The model under review builds one solid part; all positions refer to its coordinate system, in mm. Face numbers are marked on the shaded views. A direction names the side the tool comes from. Give positions to 0.01 mm unless a question says otherwise; leave off trailing zeros. Write each loop counter-clockwise with the first axis right and the second up, starting at its lowest first coordinate (ties: lowest second). Pieces come first, ordered by that corner, then holes. Notation, with made-up numbers: M 85.5,-11.5 L 96.5,-11.5 A25 ccw 96.5,3.5 Z; hole C -9.5,47 d3. An arc over 180 degrees is marked long. Write item = value, one per line. Start each with the question number.
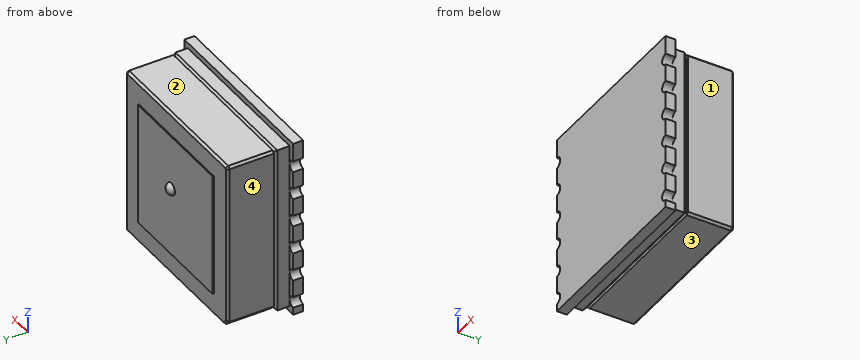
```python
from build123d import *

# Parameters (mm, degrees)
EXTRUDE1_DEPTH = 0.9
SKETCH2_W      = 15
SKETCH2_H      = 15
EXTRUDE2_DEPTH = 1.4
CHAMFER1_SIZE  = 0.3
SKETCH3_W      = 15
SKETCH3_H      = 15
EXTRUDE3_DEPTH = 4.15
CHAMFER2_SIZE  = 0.5
CHAMFER3_SIZE  = 0.2
CHAMFER4_SIZE  = 0.2
SKETCH4_R      = 0.55
EXTRUDE4_DEPTH = 0.5
FILLET1_R      = 0.5
SKETCH5_W      = 11
SKETCH5_H      = 11
EXTRUDE5_DEPTH = 0.1


with BuildPart() as part:
    # Sketch1 → Extrude1 (new body)
    with BuildSketch(Plane(origin=(0, 0, 0), x_dir=(1, 0, 0), z_dir=(0, 1, 0))):
        with BuildLine():
            Line((8, 6.35), (8, 4.81))
            ThreePointArc((8, 4.81), (7.5, 4.31), (8, 3.81))
            Line((8, 3.81), (8, 2.27))
            ThreePointArc((8, 2.27), (7.5, 1.77), (8, 1.27))
            Line((8, 1.27), (8, -0.27))
            ThreePointArc((8, -0.27), (7.5, -0.77), (8, -1.27))
            Line((8, -1.27), (8, -2.81))
            ThreePointArc((8, -2.81), (7.5, -3.31), (8, -3.81))
            Line((8, -3.81), (8, -5.35))
            ThreePointArc((8, -5.35), (7.5, -5.85), (8, -6.35))
            Line((8, -6.35), (8, -8))
            Line((8, -8), (-8, -8))
            Line((-8, -8), (-8, -6.35))
            ThreePointArc((-8, -6.35), (-7.5, -5.85), (-8, -5.35))
            Line((-8, -5.35), (-8, -3.81))
            ThreePointArc((-8, -3.81), (-7.5, -3.31), (-8, -2.81))
            Line((-8, -2.81), (-8, -1.27))
            ThreePointArc((-8, -1.27), (-7.5, -0.77), (-8, -0.27))
            Line((-8, -0.27), (-8, 1.27))
            ThreePointArc((-8, 1.27), (-7.5, 1.77), (-8, 2.27))
            Line((-8, 2.27), (-8, 3.81))
            ThreePointArc((-8, 3.81), (-7.5, 4.31), (-8, 4.81))
            Line((-8, 4.81), (-8, 6.35))
            ThreePointArc((-8, 6.35), (-7.5, 6.85), (-8, 7.35))
            Line((-8, 7.35), (-8, 8))
            Line((-8, 8), (8, 8))
            Line((8, 8), (8, 7.35))
            ThreePointArc((8, 7.35), (7.5, 6.85), (8, 6.35))
        make_face()
    extrude(amount=EXTRUDE1_DEPTH)

    # Sketch2 → Extrude2 (add)
    with BuildSketch(Plane(origin=(0, 0.9, 0), x_dir=(1, 0, 0), z_dir=(0, 1, 0))):
        Rectangle(SKETCH2_W, SKETCH2_H)
    extrude(amount=EXTRUDE2_DEPTH)

    # Chamfer1
    chamfer1_edges = [part.edges().sort_by_distance(p)[0] for p in [
        (-7.5, 2.3, 0),
        (0, 2.3, 7.5),
        (7.5, 2.3, 0),
        (0, 2.3, -7.5),
    ]]
    chamfer(chamfer1_edges, length=CHAMFER1_SIZE)

    # Sketch3 → Extrude3 (add)
    with BuildSketch(Plane(origin=(0, 2.3, 0), x_dir=(1, 0, 0), z_dir=(0, 1, 0))):
        Rectangle(SKETCH3_W, SKETCH3_H)
    extrude(amount=EXTRUDE3_DEPTH)

    # Chamfer2
    chamfer2_edges = [part.edges().sort_by_distance(p)[0] for p in [
        (-7.5, 4.375, -7.5),
    ]]
    chamfer(chamfer2_edges, length=CHAMFER2_SIZE)

    # Chamfer3
    chamfer3_edges = [part.edges().sort_by_distance(p)[0] for p in [
        (-7.5, 4.375, 7.5),
        (7.5, 4.375, 7.5),
        (7.5, 4.375, -7.5),
    ]]
    chamfer(chamfer3_edges, length=CHAMFER3_SIZE)

    # Chamfer4
    chamfer4_edges = [part.edges().sort_by_distance(p)[0] for p in [
        (-7.5, 6.45, 0.15),
        (-7.25, 6.45, -7.25),
        (0.15, 6.45, -7.5),
        (7.5, 6.45, 0),
        (0, 6.45, 7.5),
        (-7.4, 6.45, 7.4),
        (7.4, 6.45, 7.4),
        (7.4, 6.45, -7.4),
    ]]
    chamfer(chamfer4_edges, length=CHAMFER4_SIZE)

    # Sketch4 → Extrude4 (add)
    with BuildSketch(Plane(origin=(0, 6.45, 0), x_dir=(1, 0, 0), z_dir=(0, 1, 0))):
        with Locations(Location((0.6, -0.63, 0), (0, 0, 270))):
            Circle(SKETCH4_R)
    extrude(amount=EXTRUDE4_DEPTH)

    # Fillet1
    fillet1_edges = [part.edges().sort_by_distance(p)[0] for p in [
        (0.6, 6.95, 0.08),
    ]]
    fillet(fillet1_edges, radius=FILLET1_R - 0.0001)  # a hair under: the kernel refuses the full size

    # Sketch5 → Extrude5 (add)
    with BuildSketch(Plane(origin=(0, 6.45, 0), x_dir=(1, 0, 0), z_dir=(0, 1, 0))):
        Rectangle(SKETCH5_W, SKETCH5_H)
    extrude(amount=EXTRUDE5_DEPTH)


solid = part.part
```
Item 1: We need section C-C, the plane z = -1. Write out the cut boundary in (x, y), and give its area (3 significant figures).
Item 2: For the marked faces 1, 2, 3 and 4, list the 3-axis set-ups (+Z, -Z, +X, -X, +Y, -Y) from which the entire face can be reached by the end or side of a thin tool; tool diameter is ignored.
Item 3: We need section B-B, the plane x = 7. Write out the cut boundary in (y, z), and give its area (3 significant figures).
Item 4: Clearance check with flat-ended pins moving along their axes: P1, Ø2, axis at x = 1.5, z = -5, coming from the +Y side; P2, Ø0.6, axis at x = -8, z = -6, coming from the +Y side; P3, Ø1.2, axis at x = -3, y = 5, coming from the -Z side. State where each tip first meets the part, or that it passes through.
Item 5: We need section A-A, the plane y = 5.25. Write out the cut boundary in (x, z).
Item 6: We need section D-D, the plane x = -0.5. Write out the cut boundary in (y, z), and give its area (3 significant figures).
Item 7: To check wall thickness, follow probe 1 along Y at (x, z) = (-1, -3.5); probe 2 along Y at (x, z) = (6.75, -1.25); probe 3 along Z at (x, y) = (-6.75, 1.75). State the ranges of each line that lie inside material, in increasing order. Write a range as [from, to].
Worked out:
q1.outline = M -8,0 L 8,0 L 8,0.9 L 7.5,0.9 L 7.5,2 L 7.2,2.3 L 7.5,2.3 L 7.5,6.25 L 7.3,6.45 L 5.5,6.45 L 5.5,6.55 L -5.5,6.55 L -5.5,6.45 L -7.3,6.45 L -7.5,6.25 L -7.5,2.3 L -7.2,2.3 L -7.5,2 L -7.5,0.9 L -8,0.9 Z
q1.area = 98.6 mm²
q2.face_1 = +Z, -Z, +X, +Y
q2.face_2 = +Z, +X, -X, +Y
q2.face_3 = -Z, +X, -X, +Y
q2.face_4 = +Z, -Z, -X, +Y
q3.outline = M 0,-8 L 0.9,-8 L 0.9,-7.5 L 2,-7.5 L 2.3,-7.2 L 2.3,-7.5 L 6.25,-7.5 L 6.45,-7.3 L 6.45,7.3 L 6.25,7.5 L 2.3,7.5 L 2.3,7.2 L 2,7.5 L 0.9,7.5 L 0.9,8 L 0,8 Z
q3.area = 97.5 mm²
q4.P1 = 6.55
q4.P2 = 0.9
q4.P3 = -7.5
q5.outline = M -7.5,-7 L -7,-7.5 L 7.3,-7.5 L 7.5,-7.3 L 7.5,7.3 L 7.3,7.5 L -7.3,7.5 L -7.5,7.3 Z
q6.outline = M 0,-8 L 0.9,-8 L 0.9,-7.5 L 2,-7.5 L 2.3,-7.2 L 2.3,-7.5 L 6.25,-7.5 L 6.45,-7.3 L 6.45,-5.5 L 6.55,-5.5 L 6.55,5.5 L 6.45,5.5 L 6.45,7.3 L 6.25,7.5 L 2.3,7.5 L 2.3,7.2 L 2,7.5 L 0.9,7.5 L 0.9,8 L 0,8 Z
q6.area = 98.6 mm²
q7.probe_1 = [0, 6.55]
q7.probe_2 = [0, 6.45]
q7.probe_3 = [-7.5, 7.5]
